```python
from build123d import *

# Parameters (mm, degrees)
FILLET1_R = 0.75


with BuildPart() as part:
    # Sketch1 → Revolve1 (revolve)
    with BuildSketch(Plane(origin=(0, 0, 0), x_dir=(0, 0, -1), z_dir=(1, 0, 0)), mode=Mode.PRIVATE) as revolve1_sk:
        Polygon((2.7, 0), (2.7, -15), (2, -15), (2, -18), (5.1, -18), (5.1, -3.5), (7.5, -3.5), (7.5, 0), align=None)
    revolve(revolve1_sk.sketch.rotate(Axis((0, 0, 0), (0, -1, 0)), 180), axis=Axis((0, 0, 0), (0, -1, 0)))

    # Fillet1
    fillet1_edges = [part.edges().sort_by_distance(p)[0] for p in [
        (0, 0, -7.5),
        (0, -3.5, -7.5),
        (0, -18, -5.1),
    ]]
    fillet(fillet1_edges, radius=FILLET1_R)


solid = part.part
```
Could you check a few things on this model? Use its own coordinates, in mm. A direction names the side the tool comes from. Coordinates: 2 decimals unless noted, no trailing zeros. Write each loop counter-clockwise with the first axis right and the second up, starting at its lowest first coordinate (ties: lowest second). Pieces come first, ordered by that corner, then holes. Notation, with made-up numbers: (-2.5, -22.75) -> (2.5, -22.75) arc R6 ccw to (2.5, -16.75) -> close; hole circle Ø6 at (70, 20.5). An arc over 180 degrees is marked (long way). Return JSON: item names as keys, results as strings.
(1) Imagine slicing it at C-C, the plane y = -1.25. Please give me the cut outline in (x, z), then the cut area to 3 significant figures.
Numbers:
{"outline": "circle Ø15 at (0, 0); hole circle Ø5.4 at (0, 0)", "area": "154 mm2"}
(2) Which directions (+Z, -Z, +X, -X, +Y, -Y) give clear straight access to the entire face, cutting with the end or side of a thin tool? Please do faces 5 (the flat face through (0, 0, 3)), 6 (the flat face through (-5, -3.5, -2)), 7 (the cylindrical face through (1.643, -7.605, -2.143)).
Numbers:
{"face 5": "+Z, -Z, +X, -X, +Y", "face 6": "-Y", "face 7": "+Y"}
(3) I'm going to push flat-ended pins straight in: pin 1 (4.5 mm diameter, centred on x = 0, z = 0, fed in from +Y); pin 2 (1.5 mm diameter, centred on x = -5, y = -12, fed in from +Z); pin 3 (2 mm diameter, centred on y = -5.5, z = -1.5, fed in from -X). Where does each tip first touch, or does it pass through?
Numbers:
{"pin 1": "stops at y = -15", "pin 2": "stops at z = 2.82", "pin 3": "stops at x = -5.08"}
(4) I need wall thicknesses on L1, parallel to X at y = -16.45, z = 0; L2, parallel to X at y = -6, z = 0; L3, parallel to Y at x = 5.75, z = 1. Which ranges of each line are inside material? Lowest first, please.
Numbers:
{"L1": "x = -5.1 to -2, 2 to 5.1", "L2": "x = -5.1 to -2.7, 2.7 to 5.1", "L3": "y = -3.5 to 0"}
(5) We'd pull the mould along X, two halves only. Please class faces 1 (the cylindrical face through (-1.532, -10.279, 4.864)), 2 (the flat face through (1, -15, -2)), 3 (the flat face through (2, -18, -1)), 4 (the cylindrical face through (2, -17, 0)): +X half, -X half, draft (parallel to the pull), parting line (faces both ways), or undercut.
Numbers:
{"face 1": "parting line", "face 2": "undercut", "face 3": "draft", "face 4": "undercut"}
(6) Imagine slicing it at A-A, the plane x = 0. Please give me the cut outline in (y, z), then the cut area to 3 significant figures.
Numbers:
{"outline": "(-18, -4.35) arc R0.75 ccw to (-17.25, -5.1) -> (-3.5, -5.1) -> (-3.5, -6.75) arc R0.75 ccw to (-2.75, -7.5) -> (-0.75, -7.5) arc R0.75 ccw to (0, -6.75) -> (0, -2.7) -> (-15, -2.7) -> (-15, -2) -> (-18, -2) -> close; (-18, 2) -> (-15, 2) -> (-15, 2.7) -> (0, 2.7) -> (0, 6.75) arc R0.75 ccw to (-0.75, 7.5) -> (-2.75, 7.5) arc R0.75 ccw to (-3.5, 6.75) -> (-3.5, 5.1) -> (-17.25, 5.1) arc R0.75 ccw to (-18, 4.35) -> close", "area": "107 mm2"}
(7) Imagine slicing it at B-B, the plane z = 0. Please give me the cut outline in (x, y).
Numbers:
{"outline": "(-7.5, -2.75) arc R0.75 ccw to (-6.75, -3.5) -> (-5.1, -3.5) -> (-5.1, -17.25) arc R0.75 ccw to (-4.35, -18) -> (-2, -18) -> (-2, -15) -> (-2.7, -15) -> (-2.7, 0) -> (-6.75, 0) arc R0.75 ccw to (-7.5, -0.75) -> close; (2, -18) -> (4.35, -18) arc R0.75 ccw to (5.1, -17.25) -> (5.1, -3.5) -> (6.75, -3.5) arc R0.75 ccw to (7.5, -2.75) -> (7.5, -0.75) arc R0.75 ccw to (6.75, 0) -> (2.7, 0) -> (2.7, -15) -> (2, -15) -> close"}
(8) Imagine slicing it at D-D, the plane y = -13.75. Please give me the cut outline in (x, z).
Numbers:
{"outline": "circle Ø10.2 at (0, 0); hole circle Ø5.4 at (0, 0)"}
